CAD build for the part. Positions are in the model's coordinates, mm. A direction names the side the tool comes from. Round coordinates to 2 decimals unless told otherwise and drop trailing zeros. Loops run counter-clockwise (first coordinate to the right, second up) from the corner with the lowest first, then second, coordinate; pieces in that order, holes last. Notation, with made-up numbers: (25, 34.5) - (45, 34.5) arc R16 ccw to (45, 65.5) - close; hole circle Ø11 at (-12.75, 28.5). An arc over 180 degrees is marked (long way). One line per question, with ' | ' between items.
Autodesk Inventor part; units mm, degrees
ref_plane "Work Plane1" through (8, 0, 0) normal (1, 0, 0) x (0, 1, 0)
ref_plane "XZ Plane" through (0, 0, 0) normal (0, 1, 0) x (-1, 0, 0)
ref_plane "XY Plane" through (0, 0, 0) normal (0, 0, 1) x (1, 0, 0)
sketch "Sketch1" plane through (0, 0, 0) normal (0, 1, 0) x (-1, 0, 0)
  circle A0 centre (0, 0) radius 3
  dimension "d0" = 6
extrude "Extrusion1" add sketch "Sketch1" along normal blind 50
ref_plane "Work Plane1" through (8, 0, 0) normal (1, 0, 0) x (0, 1, 0)
sketch "Sketch2" plane through (8, 0, 0) normal (1, 0, 0) x (0, 1, 0)
  line L0 (0, -3) -> (50, -3)
  line L1 (0, 3) -> (50, 3)
  line L2 (40, -3) -> (20, -3)
  line L3 (20, -3) -> (20, 3)
  line L4 (20, 3) -> (40, 3)
  line L5 (40, 3) -> (40, -3)
  line L6 (20, -3) -> (10, -3)
  line L7 (10, -3) -> (10, 3)
  line L8 (10, 3) -> (20, 3)
  line L9 (20, 3) -> (20, -3)
  line L10 (0, -3) -> (0, 3)
  line L11 (50, -3) -> (50, 3)
  point P0 (0, 0)
  point P1 (20, -3)
  point P2 (20, 3)
  point P3 (10, 3)
  point P4 (10, -3)
  point P5 (40, 3)
  point P6 (20, -3)
  dimension "d4" = 20
  dimension "d5" = 10
  dimension "d7" = 10
  dimension "d19" = 30
extrude "Extrusion2" add sketch "Sketch2" against normal blind 14 contours L7 L1 L3 L0 | L3 L1 L5 L0
sketch "Sketch6" plane through (8, 10, -3) normal (0, 0, -1) x (-1, 0, 0)
  circle A0 centre (8.5023, 25) radius 3
  circle A1 centre (8.5023, 5) radius 3
  line L0 (8, 30) -> (14, 30)
  line L1 (8, 0) -> (14, 0)
  point P0 (8, -10)
  dimension "d36" = 6
  dimension "d37" = 6
  dimension "d38" = 0
  dimension "d39" = 5
  dimension "d40" = 5
extrude "Extrusion5" cut sketch "Sketch6" against normal blind 3
sketch "Sketch7" plane through (8, 10, -3) normal (0, 0, -1) x (-1, 0, 0)
  line L0 (14, 30) -> (14, 0)
  line L1 (8, 30) -> (14, 30)
  point P0 (8, -10)
  point P1 (8, 15)
  dimension "d43" = 6
  dimension "d44" = 15
hole "Hole2" at (0, 25, -3) direction (0, 0, 1) diameter 4.917 end through all
sketch "Sketch9" plane through (-6, 40, -3) normal (0, 1, 0) x (1, 0, 0)
  circle A0 centre (6, -3) radius 5.831
  circle A1 centre (6, -3) radius 3
  circle A2 centre (6, -3) radius 10
  dimension "d54" = 11.662
  dimension "d55" = 20
extrude "Extrusion7" cut sketch "Sketch9" against normal blind 40 contours A2
properties part number "slider"
(1) Cut at A-A, the plane y = 25. Write the cut outline in (x, z), then the cut area to 3 significant figures.
Results found:
outline: (-5, -3) - (-2.46, -3) - (-2.46, 3) - (-5, 3) arc R5.83 ccw to start; (2.46, -3) - (5, -3) arc R5.83 ccw to (5, 3) - (2.46, 3) - close | area: 37.2 mm²
(2) Tool access for faces 1 (the face through (0.15, 12.07, -1.52)), 2 (the face through (4, 40, 0)), 3 (the face through (4, 10, 0)): list every direction of +Z, -Z, +X, -X, +Y, -Y with a clear straight run to the whole face (end or side of a thin tool).
Results found:
face 1: -Z | face 2: +X, +Y | face 3: +X, -Y
(3) Probe L1, parallel to Y at x = -2, z = -1; L2, parallel to Y at x = 0, z = 1.4; L3, parallel to Y at x = -1.75, z = -1. List the from-to ranges inside material, lowest first.
Results found:
L1: y = 0 to 12.4, 17.6 to 23.57, 26.43 to 32.4, 37.6 to 50 | L2: y = 0 to 22.54, 27.46 to 50 | L3: y = 0 to 12.27, 17.73 to 23.27, 26.73 to 32.27, 37.73 to 50
(4) Cut at C-C, the plane z = 2. Write the cut outline in (x, y), then the cut area to 3 significant figures.
Results found:
outline: (-5.48, 10) - (-2.24, 10) - (-2.24, 0) - (2.24, 0) - (2.24, 10) - (5.48, 10) - (5.48, 40) - (2.24, 40) - (2.24, 50) - (-2.24, 50) - (-2.24, 40) - (-5.48, 40) - close; hole circle Ø4.92 at (0, 25) | area: 399 mm²
(5) Drop flat-ended pins along their axis: P1, Ø1, axis at x = -1, y = 7, coming from the +Z side; P2, Ø5, axis at x = -0.5, y = 15, coming from the -Z side; P3, Ø1.5, axis at x = -4, z = -1, coming from the -Y side. Give the stop position or say it passes through.
Results found:
P1: stops at z = 2.96 | P2: stops at z = 0 | P3: stops at y = 10
(6) Cut at D-D, the plane y = 15. Write the cut outline in (x, z), then the cut area to 3 significant figures.
Results found:
outline: (-5, -3) - (-3.5, -3) - (-3.5, 0) - (2.5, 0) - (2.5, -3) - (5, -3) arc R5.83 ccw to (5, 3) - (-5, 3) arc R5.83 ccw to start | area: 48.7 mm²
(7) Two-plate mould, pull along X, no slides. Class faces 4 (the face through (3, 5, 0)), 5 (the face through (-0.112, 37.974, -1.521)), 6 (the face through (-5.83, 25.21, -0.04)), 7 (the face through (0, 15, 0)): released by +X, released by -X, zero draft, split by the parting line, or undercut.
Results found:
face 4: split by the parting line | face 5: undercut | face 6: released by -X | face 7: undercut
(8) Cut at B-B, the plane x = 2. Write the cut outline in (y, z), then the cut area to 3 significant figures.
Results found:
outline: (0, -2.24) - (10, -2.24) - (10, -3) - (13.35, -3) - (13.35, 0) - (16.65, 0) - (16.65, -3) - (23.57, -3) - (23.57, 3) - (10, 3) - (10, 2.24) - (0, 2.24) - close; (26.43, -3) - (33.35, -3) - (33.35, 0) - (36.65, 0) - (36.65, -3) - (40, -3) - (40, -2.24) - (50, -2.24) - (50, 2.24) - (40, 2.24) - (40, 3) - (26.43, 3) - close | area: 232 mm²
